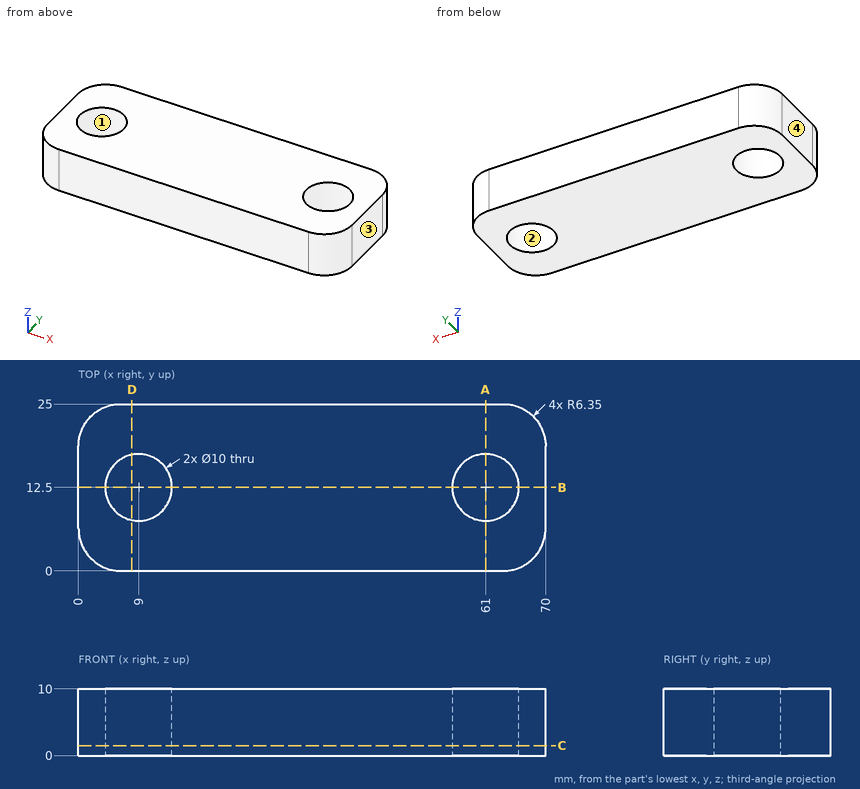
Drawing for the job (mm, zero at the part's lowest x, y, z). Give positions to 0.01 mm unless a question says otherwise; leave off trailing zeros. Order: outer loops, then holes, each group sorted by start corner. A loop starts at its lowest first (then second) coordinate and runs counter-clockwise, first axis right, second up. Notation, with made-up numbers: (86.25, 10.25) -> (92.25, 10.25) arc R16 ccw to (92.25, 39.25) -> close; hole circle Ø10 at (17, -15). An arc over 180 degrees is marked (long way). Use one line per item in the form item = value.
(1) Pull direction X, two halves, no side cores. Call the marked faces 1, 2, 3 and 4: +X half, -X half, draft (parallel to the pull), parting line (faces both ways), or undercut.
Solution:
face_1 = undercut
face_2 = undercut
face_3 = +X half
face_4 = -X half
(2) Saw through at B-B (y = 12.5). Write the cut outline in (x, z), then the cut area to 3 significant figures.
Solution:
outline = (0, 0) -> (4, 0) -> (4, 10) -> (0, 10) -> close; (14, 0) -> (56, 0) -> (56, 10) -> (14, 10) -> close; (66, 0) -> (70, 0) -> (70, 10) -> (66, 10) -> close
area = 500 mm²
(3) Drill centre lines: line 1 (Y direction, x = 61, z = 7.25); line 2 (X direction, y = 11.5, z = 0.5); line 3 (X direction, y = 14.75, z = 2.25). Where is each one in solid material? Low to high. Write a range as from..to.
Solution:
line_1 = 0..7.5, 17.5..25
line_2 = 0..4.1, 13.9..56.1, 65.9..70
line_3 = 0..4.53, 13.47..56.53, 65.47..70
(4) Saw through at C-C (z = 1.5). Write the cut outline in (x, y).
Solution:
outline = (0, 6.35) arc R6.35 ccw to (6.35, 0) -> (63.65, 0) arc R6.35 ccw to (70, 6.35) -> (70, 18.65) arc R6.35 ccw to (63.65, 25) -> (6.35, 25) arc R6.35 ccw to (0, 18.65) -> close; hole circle Ø10 at (9, 12.5); hole circle Ø10 at (61, 12.5)
(5) Flat gauge pin, fed straight in: P1, Ø12, axis at x = 8.5, y = 7, coming from the -Z side. Where does the tip first touch, or does it go through?
Solution:
P1 = 0
(6) Saw through at A-A (x = 61). Write the cut outline in (y, z), then the cut area to 3 significant figures.
Solution:
outline = (0, 0) -> (7.5, 0) -> (7.5, 10) -> (0, 10) -> close; (17.5, 0) -> (25, 0) -> (25, 10) -> (17.5, 10) -> close
area = 150 mm²
(7) Saw through at D-D (x = 8). Write the cut outline in (y, z).
Solution:
outline = (0, 0) -> (7.6, 0) -> (7.6, 10) -> (0, 10) -> close; (17.4, 0) -> (25, 0) -> (25, 10) -> (17.4, 10) -> close
